Read the model definition and answer for the solid it produces. Units are mm, in the model's axes. A direction names the side the tool comes from. Coordinates: 2 decimals unless noted, no trailing zeros. Order: outer loops, then holes, each group sorted by start corner. A loop starts at its lowest first (then second) coordinate and runs counter-clockwise, first axis right, second up. Notation, with made-up numbers: M 60,27.25 L 110,27.25 A31 ccw 110,63.25 Z; hole C -22.5,-38 d4. An arc over 180 degrees is marked long. Write each question's results on one line, items separated by ' | '.
```python
from build123d import *

# Parameters (mm, degrees)
EXTRUDE_9_DEPTH      = 5
CUT_EXTRUDE_7_DEPTH  = 2.5
SKETCH_53_R          = 3
CUT_EXTRUDE_12_DEPTH = 5
SKETCH_54_R          = 2.1
CUT_EXTRUDE_14_DEPTH = 291.088033153


with BuildPart() as part:
    # 草图51 → 凸台-拉伸9 (new body)
    with BuildSketch(Plane.XY.offset(20)):
        Polygon((198.176593222, -40.983726982), (99.565497293, 129.815701356), (-97.656694564, 129.815701356), (-196.267790492, -40.983726982), (-97.656694564, -211.78315532), (99.565497293, -211.78315532), align=None)
    extrude(amount=EXTRUDE_9_DEPTH)

    # 草图52 → 切除-拉伸7 (cut)
    with BuildSketch(Plane.XY.offset(25)):
        Polygon((-195.113089954, -40.983726982), (-97.079344294, 128.815701356), (98.988147024, 128.815701356), (197.021892683, -40.983726982), (98.988147024, -210.78315532), (97.833446486, -208.78315532), (194.712491607, -40.983726982), (97.833446486, 126.815701356), (-95.924643756, 126.815701356), (-192.803688877, -40.983726982), (-95.924643756, -208.78315532), (-97.079344294, -210.78315532), align=None)
    extrude(amount=-CUT_EXTRUDE_7_DEPTH, mode=Mode.SUBTRACT)

    # 草图53 → 切除-拉伸12 (cut)
    with BuildSketch(Plane(origin=(0, 0, 20), x_dir=(-1, 0, 0), z_dir=(0, 0, -1))):
        with Locations((-67.98, -118.86)):
            Circle(SKETCH_53_R)
        with Locations((-67.98, 117.66)):
            Circle(SKETCH_53_R)
        with Locations((67.98, 117.66)):
            Circle(SKETCH_53_R)
        with Locations((-112.33, -29.68)):
            Circle(SKETCH_53_R)
        with Locations((121.69, -29.68)):
            Circle(SKETCH_53_R)
        with Locations((-135, 0)):
            Circle(SKETCH_53_R)
        with Locations((135, 0)):
            Circle(SKETCH_53_R)
        with Locations((-122.33, 29.64)):
            Circle(SKETCH_53_R)
        with Locations((121.69, 29.64)):
            Circle(SKETCH_53_R)
        with Locations((67.98, -118.86)):
            Circle(SKETCH_53_R)
    extrude(amount=-CUT_EXTRUDE_12_DEPTH, mode=Mode.SUBTRACT)

    # 草图54 → 切除-拉伸14 (cut, through all)
    with BuildSketch(Plane.XY.offset(20)):
        with Locations((-49.045598635, -199.78315532)):
            Circle(SKETCH_54_R)
        with Locations(Location((50.954401365, -199.78315532, 0), (0, 0, 180))):
            Circle(SKETCH_54_R)
        with Locations((-49.045598635, -159.78315532)):
            Circle(SKETCH_54_R)
        with Locations(Location((50.954401365, -159.78315532, 0), (0, 0, 180))):
            Circle(SKETCH_54_R)
    extrude(amount=CUT_EXTRUDE_14_DEPTH, mode=Mode.SUBTRACT)


solid = part.part
```
(1) Straight lines are drawn through the part: line 1 (Y direction, x = -67.98, z = 23.3); line 2 (X direction, y = -138, z = 23.85); line 3 (Y direction, x = 112.33, z = 23.3). For each, find the intervals that lie inside material, in ascending order.
Conclusion:
line 1: -211.78 to -121.86, -115.86 to 114.66, 120.66 to 126.82, 128.82 to 129.82 | line 2: -140.26 to -139.1, -136.79 to 138.7, 141.01 to 142.16 | line 3: -189.67 to -187.67, -183.67 to -32.68, -26.68 to 101.71, 105.71 to 107.71
(2) Given pin 1 (1 mm diameter, centred on x = 149, z = 23.5, fed in from +Y); pin 2 (1.5 mm diameter, centred on y = -142, z = 24.5, fed in from -X), each flat-ended and moving along its own axis, determine where each tip first touches the part or whether it passes through.
Conclusion:
pin 1: y = 45.06 | pin 2: x = -138.38
(3) The mould has two halves that part along X. Classify faces 3 (the flat face through (145.595, -126.058, 23.768)), 4 (the flat face through (-147.65, -125.19, 22.46)), 5 (the flat face through (-2, -39, 20)): pulls with the +X half, pulls with the -X half, needs draft (parallel to the pull), parting line crosses it, or undercut.
Conclusion:
face 3: undercut | face 4: pulls with the -X half | face 5: needs draft
(4) The part is cut by section B-B, the plane x = -170. Write down the section's boundary in (y, z).
Conclusion:
outline: M -86.48,20 L 4.51,20 L 4.51,25 L 2.51,25 L 2.51,22.5 L -1.49,22.5 L -1.49,25 L -80.48,25 L -80.48,22.5 L -84.48,22.5 L -84.48,25 L -86.48,25 Z
(5) The part is cut by section C-C, the plane z = 23.95. Count the separate pieces of the cut face and the enclosed holes in it, then the cut area to 3 significant figures.
Conclusion:
separate pieces: 1 | enclosed holes: 15 | area: 98,800 mm²
(6) The part is cut by section A-A, the plane y = 68.5. Write down the section's boundary in (x, z), then the cut area to 3 significant figures.
Conclusion:
outline: M -133.06,20 L 134.97,20 L 134.97,25 L 133.81,25 L 133.81,22.5 L 131.5,22.5 L 131.5,25 L -129.59,25 L -129.59,22.5 L -131.9,22.5 L -131.9,25 L -133.06,25 Z | area: 1,330 mm²
(7) For faces 1 (the flat face through (146.95, 41.74, 23.77)), 2 (the flat face through (149.56, 43.22, 22.46)), determine the directions among +Z, -Z, +X, -X, +Y, -Y from which every point of the face is accessible in a straight line to the end or side of a thin tool.
Conclusion:
face 1: +Z | face 2: +Z, -Z, +X, +Y
